Here's the drawing with two shaded views (mm, measured from the low corner). I have some questions. Round coordinates to 2 decimals unless told otherwise and drop trailing zeros. Loops run counter-clockwise (first coordinate to the right, second up) from the corner with the lowest first, then second, coordinate; pieces in that order, holes last.
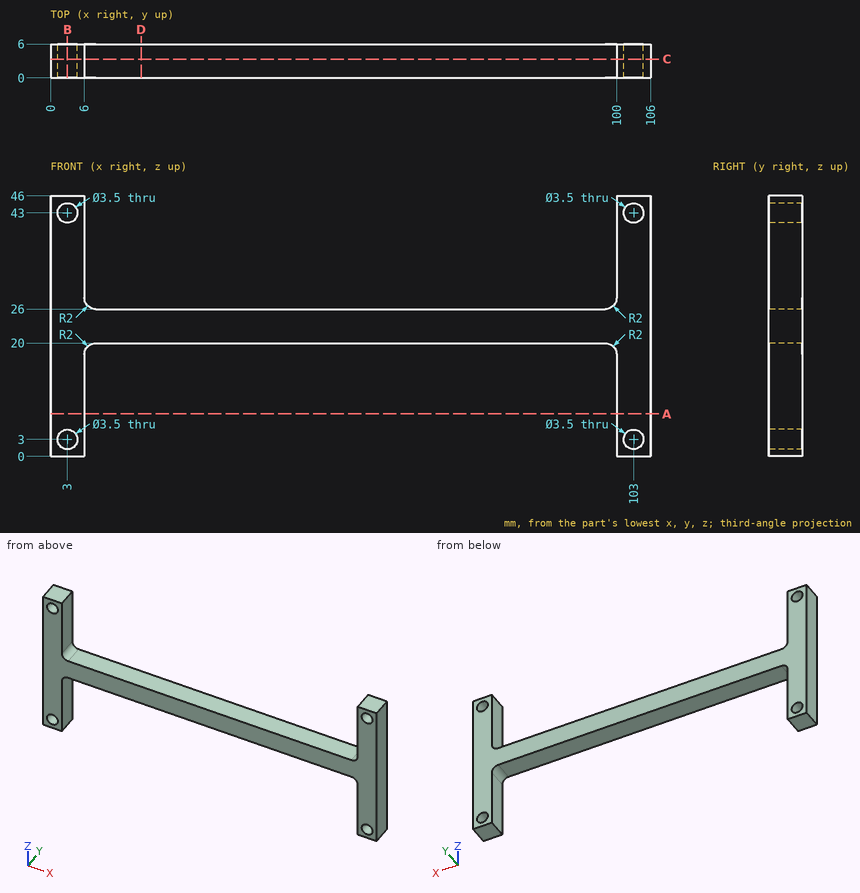
(1) If I drill on line 1 (Z direction, x = 103, y = 3.35); line 2 (X direction, y = 2.4, z = 3); line 3 (X direction, y = 1.3, z = 41), over which ranges is the centre line in solid material (lowest first)?
Worked answers:
line 1: z = 0 to 1.25, 4.75 to 41.25, 44.75 to 46
line 2: x = 0 to 1.25, 4.75 to 6, 100 to 101.25, 104.75 to 106
line 3: x = 0 to 6, 100 to 106
(2) If we section it at D-D, the plane x = 16: List the corners of the cut face in (y, z) for me, then the cut area to 3 significant figures.
Worked answers:
outline: (0, 20) - (6, 20) - (6, 26) - (0, 26) - close
area: 36.0 mm2
(3) If we section it at B-B, the plane x = 3: List the corners of the cut face in (y, z) for me.
Worked answers:
outline: (0, 0) - (6, 0) - (6, 1.25) - (0, 1.25) - close; (0, 4.75) - (6, 4.75) - (6, 41.25) - (0, 41.25) - close; (0, 44.75) - (6, 44.75) - (6, 46) - (0, 46) - close
(4) If we section it at C-C, the plane y = 3.35: List the corners of the cut face in (x, z) for me.
Worked answers:
outline: (0, 0) - (6, 0) - (6, 18) arc R2 cw to (8, 20) - (98, 20) arc R2 cw to (100, 18) - (100, 0) - (106, 0) - (106, 46) - (100, 46) - (100, 28) arc R2 cw to (98, 26) - (8, 26) arc R2 cw to (6, 28) - (6, 46) - (0, 46) - close; hole circle Ø3.5 at (3, 3); hole circle Ø3.5 at (3, 43); hole circle Ø3.5 at (103, 3); hole circle Ø3.5 at (103, 43)
(5) If we section it at A-A, the plane z = 7.5: List the corners of the cut face in (x, y) for me, then the cut area to 3 significant figures.
Worked answers:
outline: (0, 0) - (6, 0) - (6, 6) - (0, 6) - close; (100, 0) - (106, 0) - (106, 6) - (100, 6) - close
area: 72.0 mm2
(6) Will these pins go through, and if not, where does the flat tip stop? P1, Ø12, axis at x = 20, z = 37, coming from the +Y side; P2, Ø3, axis at x = 66, y = 2, coming from the -Z side.
Worked answers:
P1: passes through
P2: stops at z = 20
